Here's the drawing with two shaded views (mm, measured from the low corner). I have some questions. Round coordinates to 2 decimals unless told otherwise and drop trailing zeros. Write each loop counter-clockwise with the first axis right and the second up, starting at its lowest first coordinate (ties: lowest second). Pieces come first, ordered by that corner, then holes. Notation, with made-up numbers: (-39, -33.5) - (-34, -33.5) arc R7 cw to (-34, -24.5) - close; hole circle Ø8 at (22, -10.75). An arc over 180 degrees is marked (long way). Return JSON: item names as keys, results as strings. Group by question number.
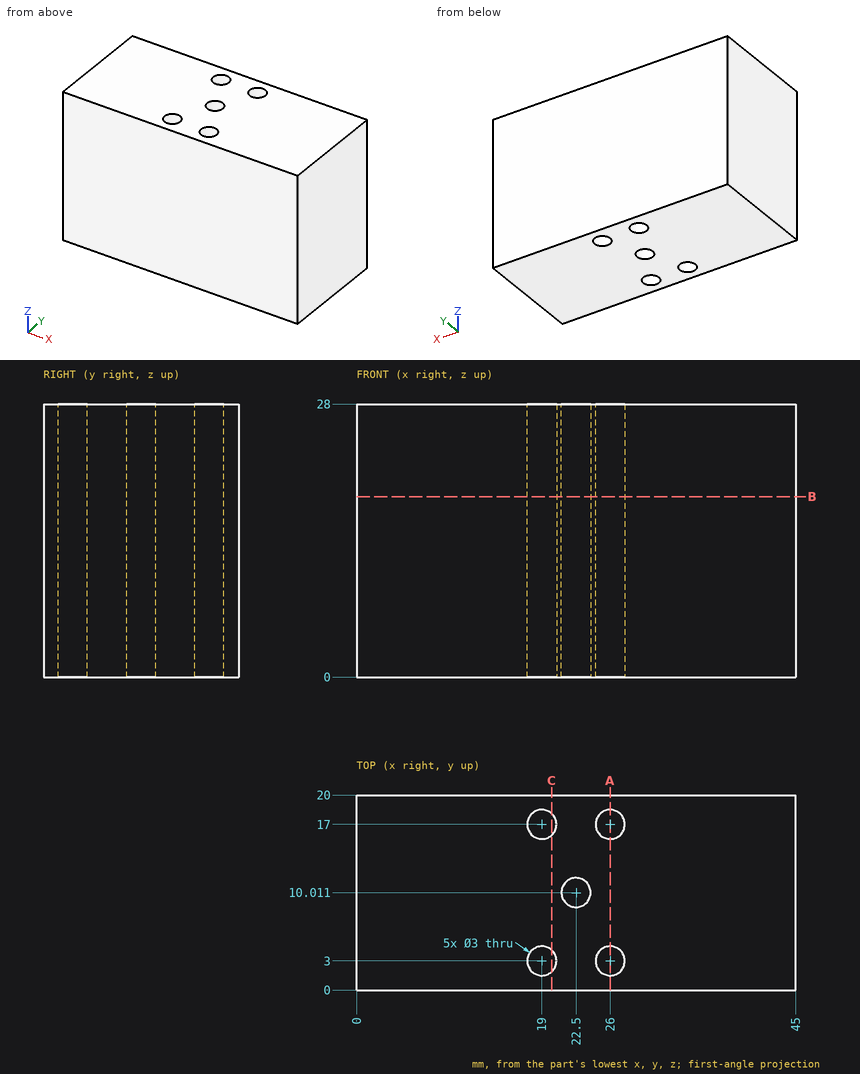
1) I need wall thicknesses on line 1 along Y through (x, z) = (19, 20.5); line 2 along Y through (x, z) = (22.5, 14); line 3 along X through (y, z) = (17.5, 20.5) (1 decimal). Which ranges of each line are inside material? Lowest first, please.
2) Imagine slicing it at B-B (z = 18.5). Please give me the cut outline in (x, y).
3) Will these pins go through, and if not, where does the flat tip stop? pin 1 Ø2.5 at (x, y) = (26, 17) entering from +Z; pin 2 Ø6 at (x, z) = (29, 5.5) entering from -Y.
4) Imagine slicing it at A-A (x = 26). Please give me the cut outline in (y, z).
5) Imagine slicing it at C-C (x = 20). Please give me the cut outline in (y, z), plus the area to 3 significant figures.
Results found:
{
 "1": {"line 1": "y = 0 to 1.5, 4.5 to 15.5, 18.5 to 20", "line 2": "y = 0 to 8.51, 11.51 to 20", "line 3": "x = 0 to 17.6, 20.4 to 24.6, 27.4 to 45"},
 "2": {"outline": "(0, 0) - (45, 0) - (45, 20) - (0, 20) - close; hole circle Ø3 at (19, 3); hole circle Ø3 at (19, 17); hole circle Ø3 at (22.5, 10.01); hole circle Ø3 at (26, 3); hole circle Ø3 at (26, 17)"},
 "3": {"pin 1": "passes through", "pin 2": "stops at y = 0"},
 "4": {"outline": "(0, 0) - (1.5, 0) - (1.5, 28) - (0, 28) - close; (4.5, 0) - (15.5, 0) - (15.5, 28) - (4.5, 28) - close; (18.5, 0) - (20, 0) - (20, 28) - (18.5, 28) - close"},
 "5": {"outline": "(0, 0) - (1.88, 0) - (1.88, 28) - (0, 28) - close; (4.12, 0) - (15.88, 0) - (15.88, 28) - (4.12, 28) - close; (18.12, 0) - (20, 0) - (20, 28) - (18.12, 28) - close", "area": "435 mm²"}
}
